```python
from build123d import *

# Parameters (mm, degrees)
SKETCH1_R           = 4
SKETCH1_R_2         = 2
BOSS_EXTRUDE1_DEPTH = 0.5
FILLET1_R           = 0.2
FILLET2_R           = 0.2


with BuildPart() as part:
    # Sketch1 → Boss-Extrude1 (new body)
    with BuildSketch(Plane(origin=(0, 0, 0), x_dir=(1, 0, 0), z_dir=(0, 1, 0))):
        Circle(SKETCH1_R)
        Circle(SKETCH1_R_2, mode=Mode.SUBTRACT)
    extrude(amount=BOSS_EXTRUDE1_DEPTH)

    # Fillet1
    fillet1_edges = [part.edges().sort_by_distance(p)[0] for p in [
        (-4, 0.5, 0),
    ]]
    fillet(fillet1_edges, radius=FILLET1_R)

    # Fillet2
    fillet2_edges = [part.edges().sort_by_distance(p)[0] for p in [
        (-4, 0, 0),
    ]]
    fillet(fillet2_edges, radius=FILLET2_R)


solid = part.part
```
Input: part model. Units: mm. Frame: model coordinates. Give positions to 0.01 mm unless a question says otherwise; leave off trailing zeros. Order: outer loops, then holes, each group sorted by start corner. A loop starts at its lowest first (then second) coordinate and runs counter-clockwise, first axis right, second up. Notation, with made-up numbers: M -30,29 L 14,29 A10 cw 14,46 Z; hole C 73,55 d4. An arc over 180 degrees is marked long. Return JSON: item names as keys, results as strings.
1) Section query C-C on y = 0.4. Output: boundary loops of the cut face in (x, z).
Taken from the geometry:
{"outline": "C 0,0 d7.95; hole C 0,0 d4"}
2) Line query: L1, parallel to X at y = 0.25, z = 0; L2, parallel to Z at x = 0.5, y = 0.35. Output: solid intervals per line, ascending. Write a range as [from, to].
Taken from the geometry:
{"L1": "x = [-4, -2], [2, 4]", "L2": "z = [-3.96, -1.94], [1.94, 3.96]"}
3) Mould query, pull axis Z, two halves, no side actions, for faces 1 (the face through (-0.434, 0.246, 1.952)), 2 (the face through (2, 0.5, 2)). Classes: released by +Z, released by -Z, zero draft, split by the parting line, or undercut.
Taken from the geometry:
{"face 1": "undercut", "face 2": "zero draft"}
4) Section query B-B on z = 0. Output: boundary loops of the cut face in (x, y).
Taken from the geometry:
{"outline": "M -4,0.2 A0.2 ccw -3.8,0 L -2,0 L -2,0.5 L -3.8,0.5 A0.2 ccw -4,0.3 Z; M 2,0 L 3.8,0 A0.2 ccw 4,0.2 L 4,0.3 A0.2 ccw 3.8,0.5 L 2,0.5 Z"}
5) Section query A-A on x = 0. Output: boundary loops of the cut face in (y, z), and give its area (3 significant figures).
Taken from the geometry:
{"outline": "M 0,-3.8 A0.2 ccw 0.2,-4 L 0.3,-4 A0.2 ccw 0.5,-3.8 L 0.5,-2 L 0,-2 Z; M 0,2 L 0.5,2 L 0.5,3.8 A0.2 ccw 0.3,4 L 0.2,4 A0.2 ccw 0,3.8 Z", "area": "1.97 mm2"}
